Part model, mm, in its own coordinate system. A direction names the side the tool comes from. Round coordinates to 2 decimals unless told otherwise and drop trailing zeros. Order: outer loops, then holes, each group sorted by start corner. A loop starts at its lowest first (then second) coordinate and runs counter-clockwise, first axis right, second up. Notation, with made-up numbers: M 44.5,20.5 L 53.5,20.5 A21 cw 53.5,40.5 Z; hole C 45.25,68.5 d7. An arc over 180 degrees is marked long. Write each question's results on one line, items separated by ' | '. Start each with the question number.
1. Band-saw the part on B-B, the plane x = -23. List the corners of the cut face in (y, z).
2. Drop flat-ended pins along their axis: pin 1 Ø8 at (y, z) = (10.5, 14.5) entering from -X; pin 2 Ø1 at (x, y) = (-19, 31.5) entering from -Z; pin 3 Ø2.5 at (y, z) = (-4.5, 4) entering from +X; pin 4 Ø4 at (x, z) = (-4.5, 13) entering from +Y. Give the stop position or say it passes through.
3. Two-plate mould, pull along X, no slides. Class faces 4 (the face through (20, -7, 4)), 5 (the face through (-8, 25, 0)), 6 (the face through (-0.297, -1.935, 13.497)), 7 (the face through (-0.865, 39.344, 0.246)): +X half, -X half, draft (parallel to the pull), parting line (faces both ways), or undercut.
4. Band-saw the part on A-A, the plane y = -8. List the corners of the cut face in (x, z), then the cut area to 3 significant figures.
5. Band-saw the part on C-C, the plane y = 2. List the corners of the cut face in (x, z).
6. Which spindle directions (+Z, -Z, +X, -X, +Y, -Y) get a long thin tool onto all of the face, cutting with end or side? Do faces 1 (the face through (0.2, -7.4, 16.5)), 2 (the face through (19.13, -7.6, 11.62)), 3 (the face through (-20, -7, 4)). Say none if no direction does.
7. Probe L1, parallel to X at y = 18, z = 2.5; L2, parallel to X at y = 16.5, z = 2.25; L3, parallel to Y at x = 26, z = 4.25. List the from-to ranges inside material, lowest first. Write a range as [from, to].
```python
from build123d import *

# Parameters (mm, degrees)
F2_ANGLE = 180
F4_DEPTH = 15
F7_R     = 5


with BuildPart() as f2:
    # F1 (on Front) → F2 (revolve)
    with BuildSketch(Plane.XZ):
        with BuildLine():
            Line((-39.353583, 0.5), (-39.353583, 0))
            Line((-39.353583, 0), (0, 0))
            Line((0, 0), (0, 19.2))
            ThreePointArc((0, 19.2), (-21.785284, 14.28726), (-39.353583, 0.5))
        make_face()
    revolve(axis=Axis((0, 0, 9.6), (0, 0, -1)), revolution_arc=F2_ANGLE)

    # F3 (on Front) → F4 (join)
    with BuildSketch(Plane.XZ):
        with BuildLine():
            Line((20, 0), (20, 12.140763))
            ThreePointArc((20, 12.140763), (0, 16.5), (-20, 12.140763))
            Line((-20, 12.140763), (-20, 0))
            Line((-20, 0), (20, 0))
        make_face()
    extrude(amount=F4_DEPTH)

    # F5 (on Top) → F6 (revolve, cut)
    with BuildSketch(Plane.XY):
        with BuildLine():
            Line((-13.5, -15), (0, -15))
            Line((0, -15), (0, 25))
            ThreePointArc((0, 25), (-9.545942, 21.045942), (-13.5, 11.5))
            Line((-13.5, 11.5), (-13.5, -15))
        make_face()
    revolve(axis=Axis((0, 5, 0), (0, 1, 0)), mode=Mode.SUBTRACT)

    # F7
    f7_edges = [f2.edges().sort_by_distance(p)[0] for p in [
        (-20, -7.5, 12.140763),
        (20, -7.5, 12.140763),
    ]]
    fillet(f7_edges, radius=F7_R)


solid = f2.part
```
Solution:
1) outline: M 0,0 L 31.93,0 L 31.93,0.5 A45.25 ccw 0,13.69 Z
2) pin 1: x = -26.58 | pin 2: z = 0 | pin 3: x = 20 | pin 4: y = 27.31
3) face 4: +X half | face 5: draft | face 6: undercut | face 7: parting line
4) outline: M -20,0 L -13.5,0 A13.5 cw 13.5,0 L 20,0 L 20,8.8 A5 ccw 16.74,13.49 A48.06 ccw -16.74,13.49 A5 ccw -20,8.8 Z | area: 313 mm^2
5) outline: M -39.3,0 L -13.5,0 A13.5 cw 13.5,0 L 39.3,0 L 39.3,0.5 A50.72 ccw -39.3,0.5 Z
6) face 1: +Z, -Y | face 2: +Z, +X, -Y | face 3: +Z, -Z, -X, -Y
7) L1: [-33.05, -11.57], [11.57, 33.05] | L2: [-34.08, -12.34], [12.34, 34.08] | L3: [0, 24.86]
